Geometry: final body of the model. Coordinates: model frame, mm. A direction names the side the tool comes from. Coordinates: 2 decimals unless noted, no trailing zeros. Write each loop counter-clockwise with the first axis right and the second up, starting at its lowest first coordinate (ties: lowest second). Pieces come first, ordered by that corner, then holes. Notation, with made-up numbers: (-37, 69) -> (8, 69) arc R28 ccw to (8, 99) -> close; hole circle Ø4 at (86, 87). An arc over 180 degrees is marked (long way). Answer as a JSON object with one key per item and string values. Group by question number.
```python
from build123d import *

# Parameters (mm, degrees)
F3_R     = 1.27
F4_DEPTH = 5.08


# Not quite as in the source:
# - a fillet or chamfer that OpenCascade refuses, or shapes differently, is made with other operations: its cross-section is extruded or revolved along the edge and cut away or added


with BuildPart() as f1:
    # F0 (on Front) → F1 (revolve)
    with BuildSketch(Plane.XZ):
        Polygon((-42.164, 0), (-34.544, 0), (-35.814, 50.8), (-37.314, 50.8), (-36.20275, 6.35), (-42.164, 6.35), align=None)
    revolve(axis=Axis((0, 0, 8.2894073013), (0, 0, -1)))

    # F2: fillet of radius 2.54 on 3 edges, made by hand

    # F2_s1 → F2_t2 (revolve)
    with BuildSketch(Plane.XZ):
        with BuildLine():
            ThreePointArc((-38.807043626, 6.35), (-36.9886872775, 7.1165344126), (-36.2678370041, 8.9534801655))
            Line((-36.2678370041, 8.9534801655), (-36.20275, 6.35))
            Line((-36.20275, 6.35), (-38.807043626, 6.35))
        make_face()
    revolve(axis=Axis((0, 0, 6.35), (0, 0, -1)))

    # F2_s3 → F2_t4 (revolve, cut)
    with BuildSketch(Plane.XZ):
        with BuildLine():
            ThreePointArc((-39.624, 6.35), (-41.4200512242, 5.6060512242), (-42.164, 3.81))
            Line((-42.164, 3.81), (-42.164, 6.35))
            Line((-42.164, 6.35), (-39.624, 6.35))
        make_face()
    revolve(axis=Axis((0, 0, 6.35), (0, 0, -1)), mode=Mode.SUBTRACT)

    # F2_s5 → F2_t6 (revolve, cut)
    with BuildSketch(Plane.XZ):
        with BuildLine():
            ThreePointArc((-37.2551532867, 48.4461314672), (-36.8821851711, 49.8358886527), (-35.814, 50.8))
            Line((-35.814, 50.8), (-37.314, 50.8))
            Line((-37.314, 50.8), (-37.2551532867, 48.4461314672))
        make_face()
    revolve(axis=Axis((0, 0, 50.8), (0, 0, -1)), mode=Mode.SUBTRACT)

    # F3 (on face) → F4 (cut)
    with BuildSketch(Plane(origin=(0, 0, 0), x_dir=(1, 0, 0), z_dir=(0, 0, -1))):
        with Locations((0, 38.1)):
            Circle(F3_R)
        with Locations((38.1, 0)):
            Circle(F3_R)
        with Locations((0, -38.1)):
            Circle(F3_R)
        with Locations((-38.1, 0)):
            Circle(F3_R)
    extrude(amount=-F4_DEPTH, mode=Mode.SUBTRACT)


solid = f1.part
```
Item 1: Section A-A on x = 0. Output: boundary loops of the cut face in (y, z).
Item 2: Section C-C on z = 46.5. Output: boundary loops of the cut face in (x, y), then the cut area to 3 significant figures.
Item 3: Section D-D on z = 20. Output: boundary loops of the cut face in (x, y), then the cut area to 3 significant figures.
Item 4: Mould query, pull axis Y, two halves, no side actions, for faces 4 (the flat face through (6.4, -34.2, 0)), 5 (the conical face through (7.97, -35.88, 28.42)), 6 (the flat face through (38, 0, 5.08)). Classes: +Y half, -Y half, draft (parallel to the pull), parting line (faces both ways), or undercut.
Item 5: Ray query, L1, parallel to Y at x = 0, z = 3.15; L2, parallel to X at y = -13.5, z = 41; L3, parallel to Y at x = -31, z = 3.5. Return the intervals inside material, ascending. Write a range as [from, to].
Item 6: Contact query for flat-ended pins moving along their axis: pin 1 (4 mm diameter, centred on y = 10, z = 30, fed in from +X); pin 2 (5 mm diameter, centred on y = -2, z = 6, fed in from +X); pin 3 (0.8 mm diameter, centred on x = 0, y = -38, fed in from -Z). Output: stop coordinate, or through.
Item 7: Set-up query: faces 1 (the conical face through (-33.563, 10.569, 25.756)), 2 (the flat face through (0, -38, 5.08)), 3 (the cylindrical face through (-40.22, 12.66, 1.88)). Return all of +Z, -Z, +X, -X, +Y, -Y with unobstructed straight access to the full face (end or side cutting, diameter ignored); none if empty.
Answer sheet:
{
 "1": {"outline": "(-42.16, 0) -> (-39.37, 0) -> (-39.37, 5.08) -> (-36.83, 5.08) -> (-36.83, 0) -> (-34.54, 0) -> (-35.81, 50.8) arc R2.54 ccw to (-37.26, 48.45) -> (-36.27, 8.95) arc R2.54 cw to (-38.81, 6.35) -> (-39.62, 6.35) arc R2.54 ccw to (-42.16, 3.81) -> close; (34.54, 0) -> (36.83, 0) -> (36.83, 5.08) -> (39.37, 5.08) -> (39.37, 0) -> (42.16, 0) -> (42.16, 3.81) arc R2.54 ccw to (39.62, 6.35) -> (38.81, 6.35) arc R2.54 cw to (36.27, 8.95) -> (37.26, 48.45) arc R2.54 ccw to (35.81, 50.8) -> close"},
 "2": {"outline": "circle Ø74.41 at (0, 0); hole circle Ø71.41 at (0, 0)", "area": "344 mm^2"},
 "3": {"outline": "circle Ø73.09 at (0, 0); hole circle Ø70.09 at (0, 0)", "area": "337 mm^2"},
 "4": {"face 4": "draft", "face 5": "parting line", "face 6": "undercut"},
 "5": {"L1": "y = [-42.16, -39.37], [-36.83, -34.62], [34.62, 36.83], [39.37, 42.16]", "L2": "x = [-34.52, -32.91], [32.91, 34.52]", "L3": "y = [-28.58, -15.44], [15.44, 28.58]"},
 "6": {"pin 1": "stops at x = 35.92", "pin 2": "stops at x = 42.16", "pin 3": "stops at z = 5.08"},
 "7": {"face 1": "+Z", "face 2": "-Z", "face 3": "+Z, -Z"}
}
